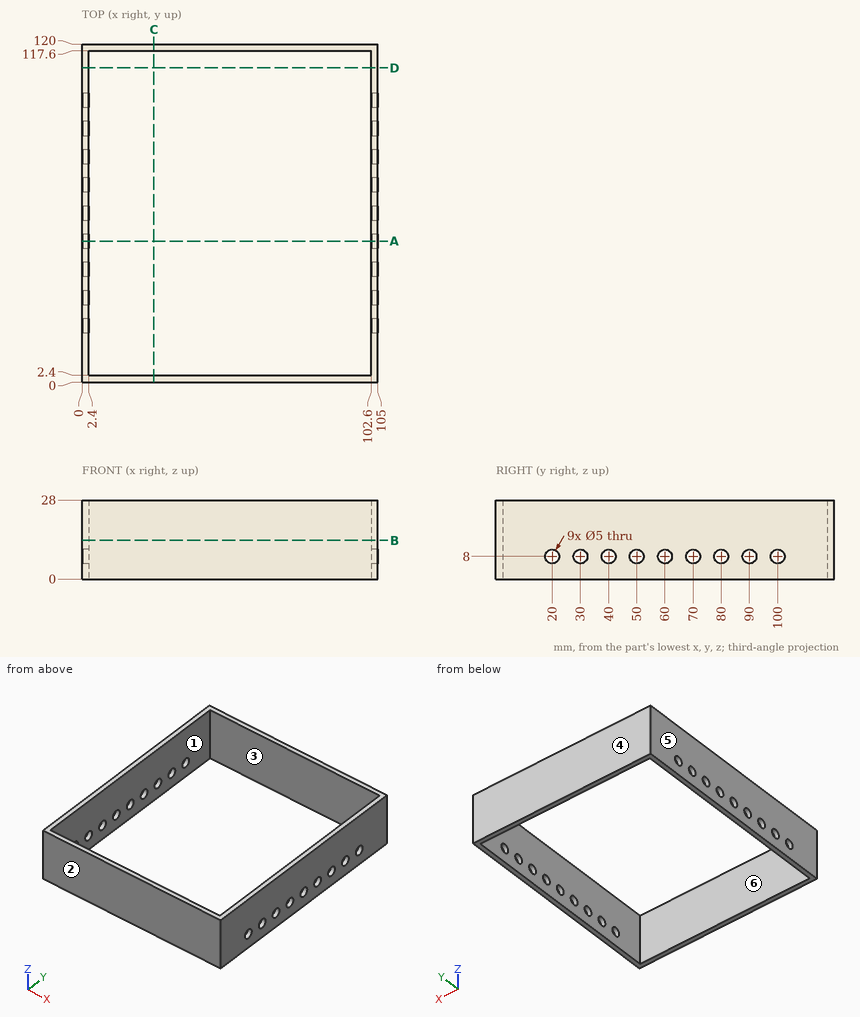
Can you work these out from the drawing? Everything is in mm from the part's minimum corner. A direction names the side the tool comes from. Round coordinates to 2 decimals unless told otherwise and drop trailing zeros. Loops run counter-clockwise (first coordinate to the right, second up) from the corner with the lowest first, then second, coordinate; pieces in that order, holes last. Notation, with made-up numbers: (67.25, -37.75) - (104.25, -37.75) arc R36 cw to (104.25, -1.75) - close; hole circle Ø5 at (-20, -0.5). An arc over 180 degrees is marked (long way). Write item = value, one per line. Start each with the question number.
(1) If we section it at B-B (z = 13.75): Please give me the cut outline in (x, y).
(2) If we section it at A-A (y = 50): Please give me the cut outline in (x, z), and give its area (3 significant figures).
(3) If I drill on probe 1 along X at (y, z) = (58, 3.75); probe 2 along Y at (x, z) = (56, 3.5); probe 3 along Z at (x, y) = (1.2, 100), over which ranges is the centre line in solid material (lowest first)? Write a range as [from, to].
(4) For P1, Ø4, axis at y = 90, z = 8, coming from the +X side; P2, Ø8, axis at y = 30, z = 8, coming from the -X side, each with a flat end and sliding along its axis, tell me the tip position at first contact or that it passes through.
(5) If we mould it in two halves opening along Y, with no side actions, what happens to the marked faces 3, 4, 5 and 6? For each: released by +Y, released by -Y, zero draft, split by the parting line, or undercut.
(6) If we section it at C-C (x = 25.5): Please give me the cut outline in (y, z).
(7) If we section it at D-D (y = 111.5): Please give me the cut outline in (x, z).
(8) For the marked faces 1 and 2, which set-ups out of +Z, -Z, +X, -X, +Y, -Y let a thin tool reach every point of the face, with its end or its side?
Ans:
q1.outline = (0, 0) - (105, 0) - (105, 120) - (0, 120) - close; hole (2.4, 2.4) - (102.6, 2.4) - (102.6, 117.6) - (2.4, 117.6) - close
q2.outline = (0, 0) - (2.4, 0) - (2.4, 5.5) - (0, 5.5) - close; (0, 10.5) - (2.4, 10.5) - (2.4, 28) - (0, 28) - close; (102.6, 0) - (105, 0) - (105, 5.5) - (102.6, 5.5) - close; (102.6, 10.5) - (105, 10.5) - (105, 28) - (102.6, 28) - close
q2.area = 110 mm²
q3.probe_1 = [0, 2.4], [102.6, 105]
q3.probe_2 = [0, 2.4], [117.6, 120]
q3.probe_3 = [0, 5.5], [10.5, 28]
q4.P1 = through
q4.P2 = 0
q5.face_3 = undercut
q5.face_4 = released by +Y
q5.face_5 = zero draft
q5.face_6 = undercut
q6.outline = (0, 0) - (2.4, 0) - (2.4, 28) - (0, 28) - close; (117.6, 0) - (120, 0) - (120, 28) - (117.6, 28) - close
q7.outline = (0, 0) - (2.4, 0) - (2.4, 28) - (0, 28) - close; (102.6, 0) - (105, 0) - (105, 28) - (102.6, 28) - close
q8.face_1 = +Z, -Z
q8.face_2 = +Z, -Z, +X, -X, -Y
